Can you work these out from the model? Positions are in its coordinate system, mm. A direction names the side the tool comes from. Give positions to 0.01 mm unless a question says otherwise; leave off trailing zeros. Loops run counter-clockwise (first coordinate to the right, second up) from the corner with the lowest first, then second, coordinate; pieces in that order, holes last. Notation, with made-up numbers: (88, 47) - (130, 47) arc R22 ccw to (130, 55) - close; hole circle Ø10 at (47, -13). An arc over 180 degrees is marked (long way). Use a Markdown table: item, result. Add a question column.
Autodesk Inventor part; units mm, degrees
ref_plane "YZ Plane" through (0, 0, 0) normal (1, 0, 0) x (0, 1, 0)
ref_plane "XZ Plane" through (0, 0, 0) normal (0, 1, 0) x (-1, 0, 0)
ref_plane "XY Plane" through (0, 0, 0) normal (0, 0, 1) x (1, 0, 0)
sketch "Sketch1" plane through (0, 0, 0) normal (0, 1, 0) x (-1, 0, 0)
  line L0 (34.29, 26.67) -> (-34.29, 26.67) construction
  line L1 (-34.29, 26.67) -> (-34.29, -26.67) construction
  line L2 (-34.29, -26.67) -> (34.29, -26.67) construction
  line L3 (34.29, -26.67) -> (34.29, 26.67) construction
  line L4 (48.006, 0) -> (-48.006, 0) construction
  line L5 (0, -37.338) -> (0, 37.338) construction
  line L6 (-31.75, -24.13) -> (-31.75, -12.7)
  line L7 (-31.75, 26.67) -> (-31.75, 22.86)
  line L8 (-34.29, -10.16) -> (-34.29, 20.32)
  line L9 (-31.75, -12.7) -> (-31.75, -12.7)
  line L10 (-31.75, 22.86) -> (-31.75, 22.86)
  line L11 (-29.21, -26.67) -> (34.29, -26.67)
  line L12 (34.29, -26.67) -> (34.29, 26.67)
  line L13 (34.29, 26.67) -> (-31.75, 26.67)
  line L14 (-31.75, -24.13) -> (-29.21, -26.67)
  line L15 (-34.29, -10.16) -> (-31.75, -12.7)
  line L16 (-34.29, 20.32) -> (-31.75, 22.86)
  circle A0 centre (20.32, -24.13) radius 1.5875
  circle A1 centre (19.05, 24.13) radius 1.5875
  circle A2 centre (-31.75, 19.05) radius 1.5875
  circle A3 centre (-31.75, -8.89) radius 1.5875
  point P0 (0, 0)
  point P1 (0, -26.67)
  point P2 (-34.29, 0)
  point P3 (-31.75, -26.67)
  point P4 (-34.29, -12.7)
  point P5 (-34.29, 22.86)
  dimension "d0" = 68.58
  dimension "d1" = 53.34
  dimension "d2" = 2.54
  dimension "d3" = 3.81
  dimension "d4" = 13.97
  dimension "d5" = 2.54
  dimension "d6" = 2.54
  dimension "d7" = 2.54
  dimension "d8" = 2.54
  dimension "d9" = 2.54
  dimension "d10" = 2.54
  dimension "d11" = 3.175
  dimension "d12" = 13.97
  dimension "d13" = 15.24
  dimension "d14" = 66.04
  dimension "d15" = 66.04
  dimension "d16" = 27.94
  dimension "d17" = 15.24
  dimension "d18" = 7.62
  dimension "d19" = 2.54
extrude "Extrusion1" add sketch "Sketch1" along normal blind 1.6002
properties part number "Arduino-Uno-r3"
1. Suppose I cut it at A-A (z = 19.05). List the corners of the cut face in (x, y) for me, and give its area (3 significant figures).
2. Suppose I cut it at B-B (y = 1.2). State how many separate pieces and enclosed holes the cut face has, and give its area (3 significant figures).
3. Will these pins go through, and if not, where does the flat tip stop? P1, Ø2.5, axis at x = 31.75, z = -8.89, coming from the -Y side; P2, Ø0.8, axis at y = 1, z = -21, coming from the +X side.
4. On a 3-axis mill with a long thin cutter (end or side, diameter ignored), from which of +Z, -Z, +X, -X, +Y, -Y can I reach the whole of each face in a straight line? I mean faces 1 (the face through (34.29, 1, 5)), 2 (the face through (31.75, 1, -18)), 3 (the face through (31.75, 1, 25)). Say none if no direction works.
5. Please list where these lines run through material, in increasing order: line 1 along Z through (x, y) = (-20.32, 0.5); line 2 along Z through (x, y) = (-19.05, 0.5); line 3 along X through (y, z) = (0.5, -15). Write a range as [from, to].
6. Suppose I cut it at C-C (z = -19). List the corners of the cut face in (x, y) for me.
7. If we mould it in two halves opening along Z, with no side actions, what happens to faces 4 (the face through (30.5, 0.79, -25.38)), 5 (the face through (0, 1.6, 0)), 6 (the face through (30.236, 0.789, 18.573)), 7 (the face through (30.284, 0.789, -8.282))? For each: released by +Z, released by -Z, zero draft, split by the parting line, or undercut.
Results below:
| question | item | result |
|---|---|---|
| 1 | outline | (-34.29, 0) - (30.16, 0) - (30.16, 1.6) - (-34.29, 1.6) - close; (33.34, 0) - (34.29, 0) - (34.29, 1.6) - (33.34, 1.6) - close |
| 1 | area | 105 mm² |
| 2 | separate pieces | 1 |
| 2 | enclosed holes | 4 |
| 2 | area | 3,570 mm² |
| 3 | P1 | through |
| 3 | P2 | x = 31.75 |
| 4 | face 1 | +Z, -Z, +X, +Y, -Y |
| 4 | face 2 | -Z, +X, +Y, -Y |
| 4 | face 3 | +Z, +X, +Y, -Y |
| 5 | line 1 | [-26.67, -25.72], [-22.54, 23.18], [25.08, 26.67] |
| 5 | line 2 | [-26.67, -25.08], [-23.18, 22.54], [25.72, 26.67] |
| 5 | line 3 | [-34.29, 31.75] |
| 6 | outline | (-34.29, 0) - (31.75, 0) - (31.75, 1.6) - (-34.29, 1.6) - close |
| 7 | face 4 | released by -Z |
| 7 | face 5 | zero draft |
| 7 | face 6 | undercut |
| 7 | face 7 | undercut |
